from build123d import *

# Parameters (mm, degrees)
SKETCH1_R           = 1.2
BOSS_EXTRUDE1_DEPTH = 13.5
SKETCH2_W           = 4
SKETCH2_H           = 4
BOSS_EXTRUDE2_DEPTH = 5.5


with BuildPart() as part:
    # Sketch1 → Boss-Extrude1 (new body, symmetric)
    with BuildSketch(Plane(origin=(0, 0, 0), x_dir=(1, 0, 0), z_dir=(0, 1, 0))):
        Circle(SKETCH1_R)
    extrude(amount=BOSS_EXTRUDE1_DEPTH, both=True)

    # Sketch2 → Boss-Extrude2 (add, symmetric)
    with BuildSketch(Plane(origin=(0, 0, 0), x_dir=(1, 0, 0), z_dir=(0, 1, 0))):
        Rectangle(SKETCH2_W, SKETCH2_H)
    extrude(amount=BOSS_EXTRUDE2_DEPTH, both=True)


solid = part.part
Verification items for the finished model (mm, model axes). A direction names the side the tool comes from. Give positions to 0.01 mm unless a question says otherwise; leave off trailing zeros. Write each loop counter-clockwise with the first axis right and the second up, starting at its lowest first coordinate (ties: lowest second). Pieces come first, ordered by that corner, then holes. Notation, with made-up numbers: M 62,28 L 116,28 A26 cw 116,42 Z; hole C 24.5,77.25 d4. An arc over 180 degrees is marked long. Use CSV: the item, a comma, the result in double quotes.
1) Cross-section at A-A (z = 0). Enter the section's corners in (x, y), plus the area to 3 significant figures.
Final values:
outline,"M -2,-5.5 L -1.2,-5.5 L -1.2,-13.5 L 1.2,-13.5 L 1.2,-5.5 L 2,-5.5 L 2,5.5 L 1.2,5.5 L 1.2,13.5 L -1.2,13.5 L -1.2,5.5 L -2,5.5 Z"
area,"82.4 mm²"
2) Cross-section at B-B (x = 0). Enter the section's corners in (y, z), plus the area to 3 significant figures.
Final values:
outline,"M -13.5,-1.2 L -5.5,-1.2 L -5.5,-2 L 5.5,-2 L 5.5,-1.2 L 13.5,-1.2 L 13.5,1.2 L 5.5,1.2 L 5.5,2 L -5.5,2 L -5.5,1.2 L -13.5,1.2 Z"
area,"82.4 mm²"
3) Access from +Z, -Z, +X, -X, +Y, -Y to the whole of each face (thin tool, end or side, straight path). Record for faces 1 (the face through (-1, -5.5, 1)), 2 (the face through (-1, 5.5, 1)), 3 (the face through (0, 0, 2)).
Final values:
face 1,"-Y"
face 2,"+Y"
face 3,"+Z, +X, -X, +Y, -Y"
4) Cross-section at D-D (z = 1.7). Enter the section's corners in (x, y), plus the area to 3 significant figures.
Final values:
outline,"M -2,-5.5 L 2,-5.5 L 2,5.5 L -2,5.5 Z"
area,"44.0 mm²"
5) Material ranges on line 1 along Y through (x, z) = (0, 1.4); line 2 along Z through (x, y) = (0.1, 7); line 3 along X through (y, z) = (6.75, -0.8), recorded low to high.
Final values:
line 1,"-5.5 to 5.5"
line 2,"-1.2 to 1.2"
line 3,"-0.89 to 0.89"
6) Cross-section at C-C (y = 6.5). Enter the section's corners in (x, z), plus the area to 3 significant figures.
Final values:
outline,"C 0,0 d2.4"
area,"4.52 mm²"
